Could you check a few things on this model? Use its own coordinates, in mm. A direction names the side the tool comes from. Give positions to 0.01 mm unless a question says otherwise; leave off trailing zeros. Write each loop counter-clockwise with the first axis right and the second up, starting at its lowest first coordinate (ties: lowest second). Pieces come first, ordered by that corner, then holes. Notation, with made-up numbers: (24.25, 43) - (62.25, 43) arc R17 cw to (62.25, 50) - close; hole circle Ø10 at (42.5, 68.5). An arc over 180 degrees is marked (long way). Answer as CSV lines item,"result". Start each with the question number.
Q1. If I drill on line 1 along Y through (x, z) = (-29, -56); line 2 along Z through (x, y) = (-41, -7); line 3 along Y through (x, z) = (-53, -37), over which ranges is the centre line in solid material (lowest first)?
Q2. Will these pins go through, and if not, where does the flat tip stop? pin 1 Ø12.5 at (x, z) = (44.5, 40.5) entering from +Y; pin 2 Ø11.5 at (x, y) = (43, -20) entering from +Z; pin 3 Ø20.5 at (y, z) = (-16.5, -40.5) entering from +X.
Q3. Imagine slicing it at C-C on y = 13. List the corners of the cut face in (x, z) for me, and give its area (3 significant figures).
Q4. We'd pull the mould along Y, two halves only. Please class faces 1 (the face through (-28, -73, -80.385)), 2 (the face through (-28, -60.81, 31)), 3 (the face through (48, -60.81, 13)): pulls with the +Y half, pulls with the -Y half, needs draft (parallel to the pull), parting line crosses it, or undercut.
Q5. On a 3-axis mill with a long thin cutter (end or side, diameter ignored), from which of +Z, -Z, +X, -X, +Y, -Y can I reach the whole of each face in a straight line? I mean faces 4 (the face through (13, -66.96, 6)), 5 (the face through (-32, -13, -61.082)), 6 (the face through (-36, 6.936, 38)). Say none if no direction works.
Q6. Imagine slicing it at A-A on x = -30.5. List the corners of the cut face in (y, z) for me, and give its area (3 significant figures).
Q7. Imagine slicing it at D-D on z = -57.5. List the corners of the cut face in (x, y) for me (3 decimals).
Q8. Imagine slicing it at B-B on z = -7.5. List the corners of the cut face in (x, y) for me.
```python
from build123d import *

# Parameters (mm, degrees)
F0_W     = 83.18023
F0_H     = 116.987984
F1_DEPTH = 25.4
F2_W     = 172.123075
F2_H     = 110.970385
F3_DEPTH = 25.4
F4_W     = 116.698637
F4_H     = 30.664335
F5_DEPTH = 25.4
F6_W     = 133.886017
F6_H     = 38.919249
F7_DEPTH = 25.4
F8_W     = 29.294722
F8_H     = 117.36656
F9_DEPTH = 25.4


with BuildPart() as f1:
    # F0 (on Right) → F1 (new body)
    with BuildSketch(Plane.YZ):
        with Locations((-25.369966, 6.922083)):
            Rectangle(F0_W, F0_H)
    extrude(amount=F1_DEPTH)

    # F2 (on Top) → F3 (join)
    with BuildSketch(Plane.XY):
        with Locations((-14.214217, -5.325139)):
            Rectangle(F2_W, F2_H)
    extrude(amount=F3_DEPTH)

    # F4 (on Front) → F5 (join)
    with BuildSketch(Plane.XZ):
        with Locations((-31.215682, -45.749648)):
            Rectangle(F4_W, F4_H)
    extrude(amount=F5_DEPTH)

    # F6 (on face) → F7 (join)
    with BuildSketch(Plane.XY.offset(25.4)):
        with Locations((-3.574874, -12.523699)):
            Rectangle(F6_W, F6_H)
    extrude(amount=F7_DEPTH)

    # F8 (on face) → F9 (join)
    with BuildSketch(Plane.XZ.offset(60.810331)):
        with Locations((-28.282989, -21.701511)):
            Rectangle(F8_W, F8_H)
    extrude(amount=F9_DEPTH)


solid = f1.part
```
Conclusion:
1,line 1,"-86.21 to -60.81, -25.4 to 0"
1,line 2,"-61.08 to -30.42, 0 to 50.8"
1,line 3,"-25.4 to 0"
2,pin 1,"y = 6.94"
2,pin 2,"z = 50.8"
2,pin 3,"x = 27.13"
3,outline,"(-100.28, 0) - (0, 0) - (0, -51.57) - (25.4, -51.57) - (25.4, 0) - (71.85, 0) - (71.85, 25.4) - (25.4, 25.4) - (25.4, 65.42) - (0, 65.42) - (0, 25.4) - (-100.28, 25.4) - close"
3,area,"6,700 mm^2"
4,face 1,"needs draft"
4,face 2,"undercut"
4,face 3,"pulls with the -Y half"
5,face 4,"+Z, -Z, +X, -Y"
5,face 5,"-Z, +X, -X, +Y"
5,face 6,"+Z, -X, +Y"
6,outline,"(-86.21, -80.38) - (-60.81, -80.38) - (-60.81, 0) - (50.16, 0) - (50.16, 25.4) - (6.94, 25.4) - (6.94, 50.8) - (-31.98, 50.8) - (-31.98, 25.4) - (-60.81, 25.4) - (-60.81, 36.98) - (-86.21, 36.98) - close; (-25.4, -61.08) - (0, -61.08) - (0, -30.42) - (-25.4, -30.42) - close"
6,area,"7,570 mm^2"
7,outline,"(-89.565, -25.4) - (27.134, -25.4) - (27.134, 0) - (-89.565, 0) - close; (-42.93, -86.21) - (-13.636, -86.21) - (-13.636, -60.81) - (-42.93, -60.81) - close"
8,outline,"(-42.93, -86.21) - (-13.64, -86.21) - (-13.64, -60.81) - (-42.93, -60.81) - close; (0, -66.96) - (25.4, -66.96) - (25.4, 16.22) - (0, 16.22) - close"
